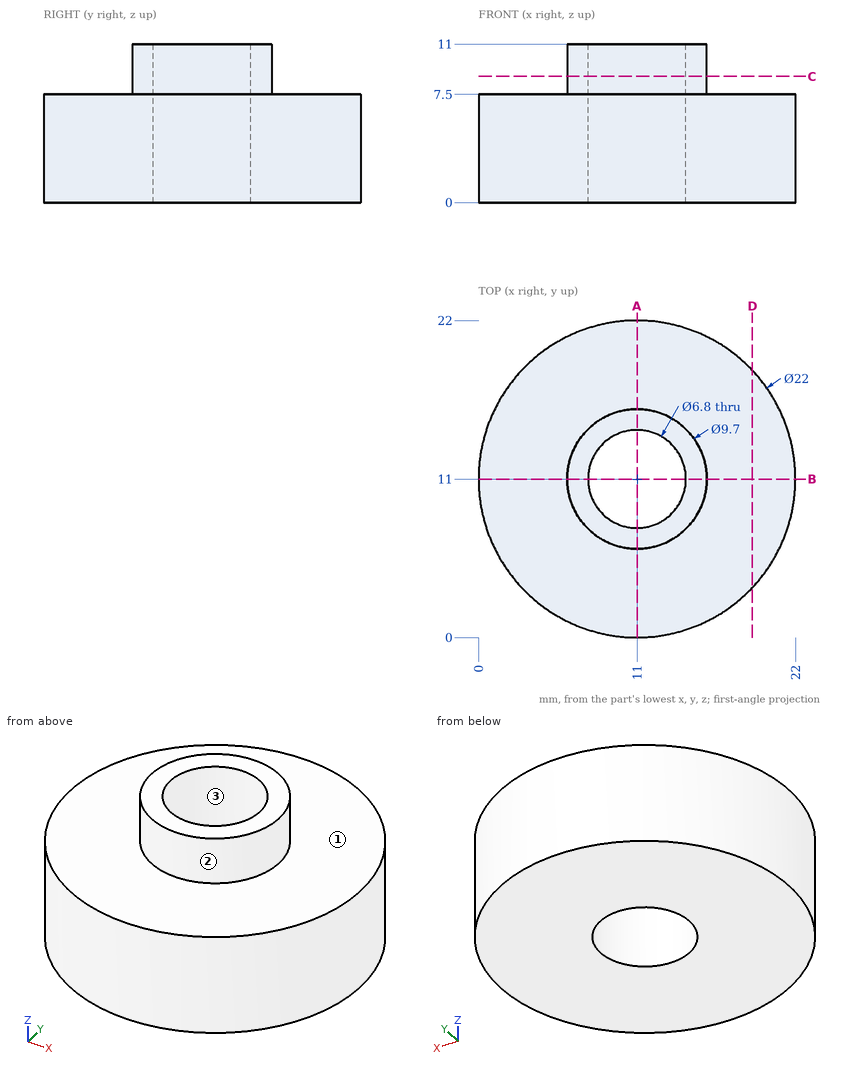
Geometry check sheet. Reference: drawing and pictorial views, mm from the part's lowest x, y, z. Give positions to 0.01 mm unless a question says otherwise; leave off trailing zeros. Write each loop counter-clockwise with the first axis right and the second up, starting at its lowest first coordinate (ties: lowest second). Pieces come first, ordered by that corner, then holes. Notation, with made-up numbers: (61, 62.5) - (109, 62.5) arc R20 ccw to (109, 96.5) - close; hole circle Ø5 at (49.25, 58). An arc over 180 degrees is marked (long way). Use a Markdown table: item, result.
Q1. Draft check along X on the marked faces 1, 2 and 3. Enter one of: pulls with the +X half, pulls with the -X half, needs draft (parallel to the pull), parting line crosses it, or undercut.
Computed:
| item | result |
|---|---|
| face 1 | needs draft |
| face 2 | parting line crosses it |
| face 3 | undercut |
Q2. Thickness scan on L1, parallel to Y at x = 11, z = 3; L2, parallel to X at y = 11, z = 9.25; L3, parallel to Z at x = 2.25, y = 7.5. Record the ranges inside material, lowest first. Write a range as [from, to].
Computed:
| item | result |
|---|---|
| L1 | y = [0, 7.6], [14.4, 22] |
| L2 | x = [6.15, 7.6], [14.4, 15.85] |
| L3 | z = [0, 7.5] |
Q3. Section check C-C, the plane z = 8.75. Enter the section's corners in (x, y).
Computed:
| item | result |
|---|---|
| outline | circle Ø9.7 at (11, 11); hole circle Ø6.8 at (11, 11) |
Q4. Section check D-D, the plane x = 19. Enter the section's corners in (y, z).
Computed:
| item | result |
|---|---|
| outline | (3.45, 0) - (18.55, 0) - (18.55, 7.5) - (3.45, 7.5) - close |
Q5. Go/stop test with flat-tipped pins: P1, Ø4, axis at x = 14.5, z = 8, coming from the +Y side; P2, Ø9, axis at x = 11, y = 11, coming from the -Z side; P3, Ø1, axis at y = 9, z = 2, coming from the +X side; P4, Ø1.5, axis at x = 16.5, z = 3.5, coming from the -Y side. Record where each tip stops, or that it passes through.
Computed:
| item | result |
|---|---|
| P1 | stops at y = 21.89 |
| P2 | stops at z = 0 |
| P3 | stops at x = 21.9 |
| P4 | stops at y = 1.08 |
Q6. Section check A-A, the plane x = 11. Enter the section's corners in (y, z).
Computed:
| item | result |
|---|---|
| outline | (0, 0) - (7.6, 0) - (7.6, 11) - (6.15, 11) - (6.15, 7.5) - (0, 7.5) - close; (14.4, 0) - (22, 0) - (22, 7.5) - (15.85, 7.5) - (15.85, 11) - (14.4, 11) - close |
